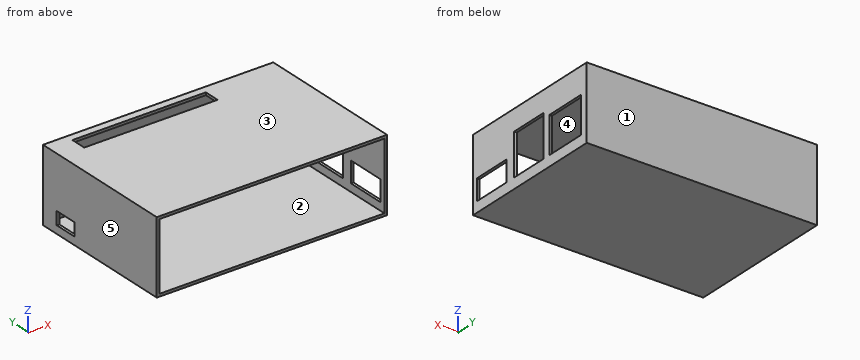
from build123d import *

# Parameters (mm, degrees)
SKETCH_1_W          = 88
SKETCH_1_H          = 58
EXTRUDE_1_DEPTH     = 28
SKETCH_2_W          = 26
SKETCH_2_H          = 56
CUT_EXTRUDE_1_DEPTH = 87
SKETCH_3_W          = 8
SKETCH_3_H          = 15
SKETCH_3_W_2        = 16
SKETCH_3_W_3        = 14
SKETCH_3_H_2        = 16
CUT_EXTRUDE_2_DEPTH = 87
SKETCH_4_W          = 28
SKETCH_4_H          = 58
EXTRUDE_2_DEPTH     = 1
SKETCH_6_W          = 51
SKETCH_6_H          = 6
CUT_EXTRUDE_4_DEPTH = 10
SKETCH_7_W          = 5
SKETCH_7_H          = 9
CUT_EXTRUDE_5_DEPTH = 10
SKETCH_8_W          = 86
SKETCH_8_H          = 26
CUT_EXTRUDE_6_DEPTH = 57


with BuildPart() as part:
    # 草图1 → 凸台-拉伸1 (new body)
    with BuildSketch(Plane.XY):
        with Locations((5.73433584, -4.901711192)):
            Rectangle(SKETCH_1_W, SKETCH_1_H)
    extrude(amount=EXTRUDE_1_DEPTH)

    # 草图2 → 切除-拉伸1 (cut)
    with BuildSketch(Plane.ZY.offset(38.26566416)):
        with Locations((14, -4.901711192)):
            Rectangle(SKETCH_2_W, SKETCH_2_H)
    extrude(amount=-CUT_EXTRUDE_1_DEPTH, mode=Mode.SUBTRACT)

    # 草图3 → 切除-拉伸2 (cut)
    with BuildSketch(Plane(origin=(49.73433584, 0, 0), x_dir=(0, 0, -1), z_dir=(1, 0, 0))):
        with Locations((-8, -24.401711192)):
            Rectangle(SKETCH_3_W, SKETCH_3_H)
        with Locations((-12, -5.401711192)):
            Rectangle(SKETCH_3_W_2, SKETCH_3_H)
        with Locations((-11, 13.098288808)):
            Rectangle(SKETCH_3_W_3, SKETCH_3_H_2)
    extrude(amount=-CUT_EXTRUDE_2_DEPTH, mode=Mode.SUBTRACT)

    # 草图4 → 凸台-拉伸2 (add)
    with BuildSketch(Plane.ZY.offset(38.26566416)):
        with Locations((14, -4.901711192)):
            Rectangle(SKETCH_4_W, SKETCH_4_H)
    extrude(amount=-EXTRUDE_2_DEPTH)

    # 草图6 → 切除-拉伸4 (cut)
    with BuildSketch(Plane.XY.offset(28)):
        with Locations((-3.76566416, 18.098288808)):
            Rectangle(SKETCH_6_W, SKETCH_6_H)
    extrude(amount=-CUT_EXTRUDE_4_DEPTH, mode=Mode.SUBTRACT)

    # 草图7 → 切除-拉伸5 (cut)
    with BuildSketch(Plane.ZY.offset(38.26566416)):
        with Locations((5.5, 12.598288808)):
            Rectangle(SKETCH_7_W, SKETCH_7_H)
    extrude(amount=-CUT_EXTRUDE_5_DEPTH, mode=Mode.SUBTRACT)

    # 草图8 → 切除-拉伸6 (cut)
    with BuildSketch(Plane.XZ.offset(33.901711192)):
        with Locations((5.73433584, 14)):
            Rectangle(SKETCH_8_W, SKETCH_8_H)
    extrude(amount=-CUT_EXTRUDE_6_DEPTH, mode=Mode.SUBTRACT)


solid = part.part
Part model, mm, in its own coordinate system. Face numbers are marked on the shaded views. A direction names the side the tool comes from. Give positions to 0.01 mm unless a question says otherwise; leave off trailing zeros. Write each loop counter-clockwise with the first axis right and the second up, starting at its lowest first coordinate (ties: lowest second). Pieces come first, ordered by that corner, then holes.
1) Two-plate mould, pull along Z, no slides. Class the marked faces 3, 4 and 5: released by +Z, released by -Z, zero draft, split by the parting line, or undercut.
Resolved:
face 3: released by +Z
face 4: undercut
face 5: zero draft
2) Pin check, flat tip, straight feed: pin 1 (3 mm diameter, centred on x = -0.5, z = 3.5, fed in from -Y). Stop position of the tip, or through.
Resolved:
pin 1: stops at y = 23.1
3) Cut at B-B on z = 16.25. Write the cut outline in (x, y).
Resolved:
outline: (-38.27, -33.9) - (-37.27, -33.9) - (-37.27, 23.1) - (48.73, 23.1) - (48.73, 21.1) - (49.73, 21.1) - (49.73, 24.1) - (-38.27, 24.1) - close; (48.73, -33.9) - (49.73, -33.9) - (49.73, -12.9) - (48.73, -12.9) - close; (48.73, 2.1) - (49.73, 2.1) - (49.73, 5.1) - (48.73, 5.1) - close
4) Cut at D-D on z = 6.5. Write the cut outline in (x, y), then the cut area to 3 significant figures.
Resolved:
outline: (-38.27, -33.9) - (-37.27, -33.9) - (-37.27, 8.1) - (-38.27, 8.1) - close; (-38.27, 17.1) - (-37.27, 17.1) - (-37.27, 23.1) - (48.73, 23.1) - (48.73, 21.1) - (49.73, 21.1) - (49.73, 24.1) - (-38.27, 24.1) - close; (48.73, -33.9) - (49.73, -33.9) - (49.73, -31.9) - (48.73, -31.9) - close; (48.73, -16.9) - (49.73, -16.9) - (49.73, -12.9) - (48.73, -12.9) - close; (48.73, 2.1) - (49.73, 2.1) - (49.73, 5.1) - (48.73, 5.1) - close
area: 147 mm2
5) Cut at A-A on x = -7. Write the cut outline in (y, z), then the cut area to 3 significant figures.
Resolved:
outline: (-33.9, 0) - (24.1, 0) - (24.1, 28) - (21.1, 28) - (21.1, 27) - (23.1, 27) - (23.1, 1) - (-33.9, 1) - close; (-33.9, 27) - (15.1, 27) - (15.1, 28) - (-33.9, 28) - close
area: 136 mm2
6) Probe L1, parallel to Z at x = -22, y = -1; L2, parallel to X at y = 19, z = 23.75; L3, parallel to X at y = 10, z = 8.5. List the from-to ranges inside material, lowest first.
Resolved:
L1: z = 0 to 1, 27 to 28
L2: x = -38.27 to -37.27, 48.73 to 49.73
L3: x = -38.27 to -37.27
7) Which spindle directions (+Z, -Z, +X, -X, +Y, -Y) get a long thin tool onto all of the face, cutting with end or side? Do the marked faces 1 and 2. Say none if no direction does.
Resolved:
face 1: +Z, -Z, +X, -X, +Y
face 2: -Y
8) Cut at C-C on y = 12. Write the cut outline in (x, z), then the cut area to 3 significant figures.
Resolved:
outline: (-38.27, 0) - (49.73, 0) - (49.73, 4) - (48.73, 4) - (48.73, 1) - (-37.27, 1) - (-37.27, 3) - (-38.27, 3) - close; (-38.27, 8) - (-37.27, 8) - (-37.27, 27) - (48.73, 27) - (48.73, 18) - (49.73, 18) - (49.73, 28) - (-38.27, 28) - close
area: 209 mm2
